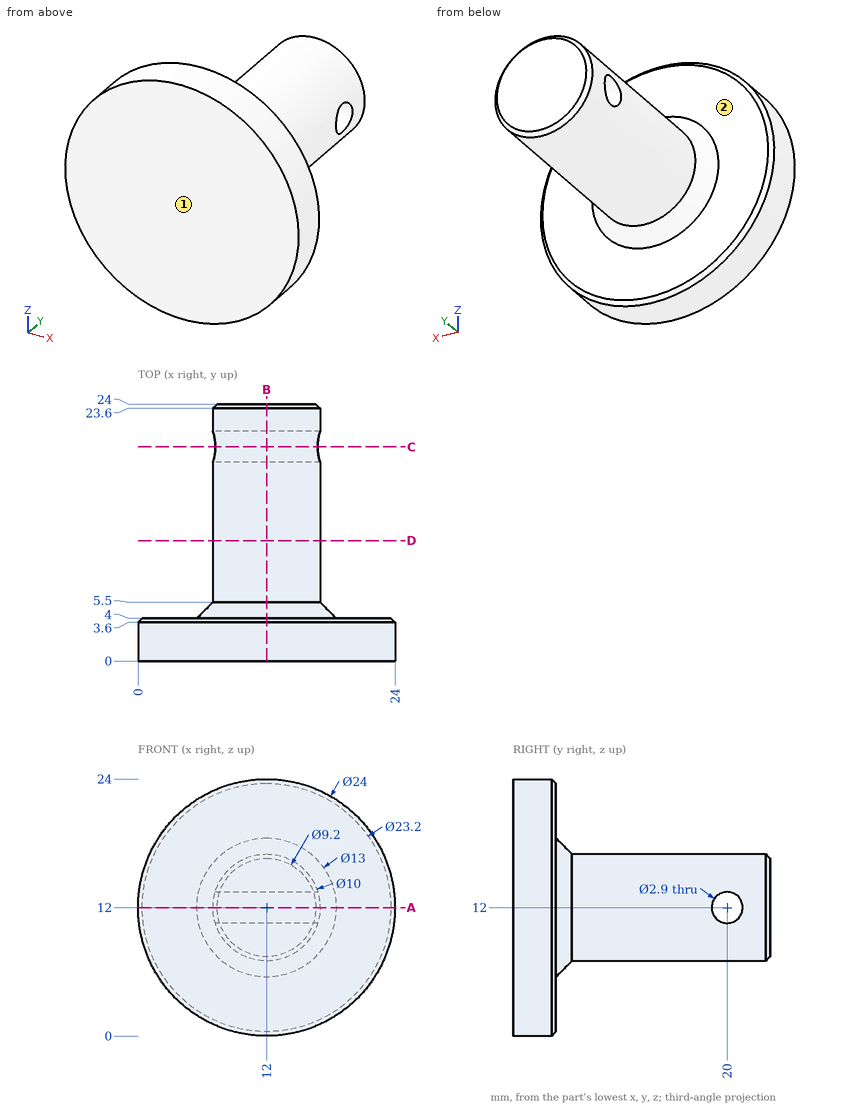
Could you check a few things on this drawing? It's one solid part, dimensions in mm from its lowest x, y, z. A direction names the side the tool comes from. Coordinates: 2 decimals unless noted, no trailing zeros. Order: outer loops, then holes, each group sorted by start corner. A loop starts at its lowest first (then second) coordinate and runs counter-clockwise, first axis right, second up. Notation, with made-up numbers: (44, 88) - (57, 88) arc R30 cw to (57, 112) - close; hole circle Ø4 at (17, 21). An arc over 180 degrees is marked (long way). One line per question, with ' | ' between items. Start each with the question number.
1. I'm going to push flat-ended pins straight in: pin 1 Ø5 at (y, z) = (19, 18) entering from -X; pin 2 Ø1 at (y, z) = (14.5, 12.5) entering from +X; pin 3 Ø12 at (x, y) = (10, 12.5) entering from -Z. Where does each tip first touch, or does it pass through?
2. If we section it at B-B (x = 12): Write out the boundary of the cut face in (y, z).
3. If we section it at D-D (y = 11.25): Write out the boundary of the cut face in (x, z), and give its area (3 significant figures).
4. Please list where these lines run through material, in increasing order: line 1 along Y through (x, z) = (9.5, 12); line 2 along Y through (x, z) = (1.75, 10.25); line 3 along Z through (x, y) = (11, 20). Write a range as [from, to].
5. Which directions (+Z, -Z, +X, -X, +Y, -Y) give clear straight access to the entire face, cutting with the end or side of a thin tool? Please do the marked faces 1 and 2.
6. If we section it at C-C (y = 20): Write out the boundary of the cut face in (x, z).
7. If we section it at A-A (z = 12): Write out the boundary of the cut face in (x, y).
Model answer:
1) pin 1: stops at x = 8.43 | pin 2: stops at x = 17 | pin 3: stops at z = 7
2) outline: (0, 0) - (3.6, 0) - (4, 0.4) - (4, 5.5) - (5.5, 7) - (23.6, 7) - (24, 7.4) - (24, 16.6) - (23.6, 17) - (5.5, 17) - (4, 18.5) - (4, 23.6) - (3.6, 24) - (0, 24) - close; hole circle Ø2.9 at (20, 12)
3) outline: circle Ø10 at (12, 12) | area: 78.5 mm²
4) line 1: y = [0, 18.55], [21.45, 24] | line 2: y = [0, 4] | line 3: z = [7.1, 10.55], [13.45, 16.9]
5) face 1: +Z, -Z, +X, -X, -Y | face 2: +Y
6) outline: (7.21, 10.55) arc R5 ccw to (16.79, 10.55) - close; (7.21, 13.45) - (16.79, 13.45) arc R5 ccw to start
7) outline: (0, 0) - (24, 0) - (24, 3.6) - (23.6, 4) - (18.5, 4) - (17, 5.5) - (17, 18.55) - (7, 18.55) - (7, 5.5) - (5.5, 4) - (0.4, 4) - (0, 3.6) - close; (7, 21.45) - (17, 21.45) - (17, 23.6) - (16.6, 24) - (7.4, 24) - (7, 23.6) - close
